Autodesk Inventor part; units mm, degrees
ref_plane "b_s_XY" through (11.5, 12, 6) normal (0, 0, 1) x (1, 0, 0)
ref_plane "b_s_YZ" through (11.5, 12, 6) normal (1, 0, 0) x (0, 1, 0)
ref_plane "b_s_ZX" through (11.5, 12, 6) normal (0, 1, 0) x (0, 0, 1)
sketch "Sketch_1" plane through (0, 0, 0) normal (0, 0, 1) x (1, 0, 0)
  line L0 (17, 0) -> (0, 0)
  line L1 (0, 18) -> (0, 6)
  line L2 (0, 6) -> (17, 6)
  line L3 (17, 6) -> (17, 18)
  line L4 (17, 18) -> (0, 18)
revolve "Revolution1" add sketch "Sketch_1" angle 360 about axis through (17, 0, 0) along (1, 0, 0)
sketch "Sketch_2" plane through (0, 0, 0) normal (0, 0, 1) x (1, 0, 0)
  line L0 (4.5, -5.8) -> (6, -5.8)
  line L1 (6, -5.8) -> (6, 30.2)
  line L2 (6, 30.2) -> (4.5, 30.2)
  line L3 (4.5, 30.2) -> (4.5, -5.8)
extrude "Extrusion1" cut sketch "Sketch_2" along normal mid plane 36
sketch "Sketch3" plane through (17, 0, 0) normal (1, 0, 0) x (0, 0, -1)
  point P0 (-12.5, 0)
hole "Hole1" at (17, 0, 12.5) direction (-1, 0, 0) diameter 5.5 depth 17 counterbore diameter 9.5 counterbore depth 12.5
sketch "Sketch4" plane through (17, 0, 0) normal (1, 0, 0) x (0, 0, -1)
  point P0 (12.5, 0)
hole "Hole2" at (17, 0, -12.5) direction (-1, 0, 0) diameter 5.5 depth 17 counterbore diameter 9.5 counterbore depth 12.5
sketch "Sketch_5" plane through (17, 0, 0) normal (1, 0, 0) x (0, 0, -1)
  line L0 (-0.75, 0) -> (0.75, 0)
  line L1 (0.75, 0) -> (0.75, 36)
  line L2 (0.75, 36) -> (-0.75, 36)
  line L3 (-0.75, 36) -> (-0.75, 0)
extrude "Extrusion2" cut sketch "Sketch_5" against normal blind 11
sketch "Sketch_6" plane through (0, 0, 0) normal (0, 0, 1) x (1, 0, 0)
  arc A0 (9.5, -6) -> (17, -14.4) centre (26.2631, 1.4189) ccw
  line L0 (17, -14.4) -> (17, 3.6)
  line L1 (17, 3.6) -> (9.5, 3.6)
  line L2 (9.5, 3.6) -> (9.5, -6)
extrude "Extrusion3" cut sketch "Sketch_6" along normal mid plane 1.5
sketch "Sketch_4" plane through (11.5, 0, 0) normal (1, 0, 0) x (0, 0, -1)
  line L0 (0, 12) -> (-18, 12)
  line L1 (-18, 12) -> (-18, 16.5)
  line L2 (-18, 16.5) -> (-6, 16.5)
  line L3 (-6, 16.5) -> (-6, 14.75)
  line L4 (-6, 14.75) -> (0, 14.75)
  line L5 (0, 14.75) -> (0, 12)
  line L6 (0, 12) -> (-18, 12)
revolve "Revolution2" cut sketch "Sketch_4" angle 360 about axis through (11.5, 12, 0) along (0, 0, -1)
sketch "Sketch_7" plane through (11.5, 0, 0) normal (1, 0, 0) x (0, 0, -1)
  line L0 (0.75, 12) -> (15.2889, 12)
  line L1 (15.2889, 12) -> (15.2889, 9.5)
  line L2 (15.2889, 9.5) -> (14.8559, 9.933)
  line L3 (14.8559, 9.933) -> (1.183, 9.933)
  line L4 (1.183, 9.933) -> (0.75, 9.5)
  line L5 (0.75, 9.5) -> (0.75, 12)
  line L6 (0.75, 12) -> (15.2889, 12)
revolve "Revolution3" cut sketch "Sketch_7" angle 360 about axis through (11.5, 12, -0.75) along (0, 0, 1)
thread "Thread1"
ref_plane "b_s_XY" through (11.5, 12, 6) normal (0, 0, 1) x (1, 0, 0)
ref_plane "b_s_YZ" through (11.5, 12, 6) normal (1, 0, 0) x (0, 1, 0)
ref_plane "b_s_ZX" through (11.5, 12, 6) normal (0, 1, 0) x (0, 0, 1)
properties part number "SSTHMR12b"
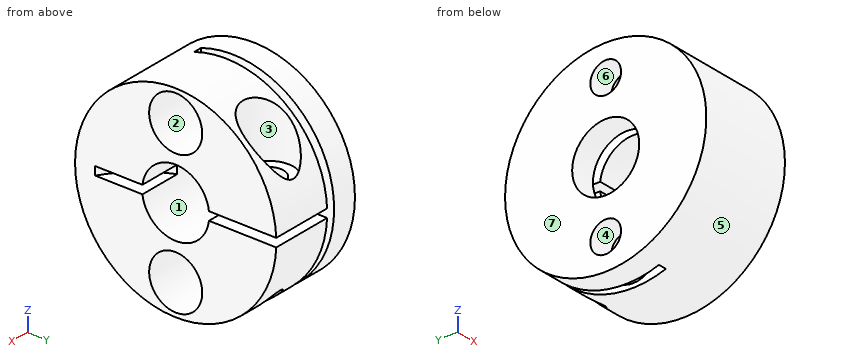
Model file for the job. Use its own axes, mm. Face numbers are marked on the shaded views. A direction names the side the tool comes from. Give positions to 0.01 mm unless a question says otherwise; leave off trailing zeros. Order: outer loops, then holes, each group sorted by start corner. A loop starts at its lowest first (then second) coordinate and runs counter-clockwise, first axis right, second up. Notation, with made-up numbers: M 85,-17.5 L 117,-17.5 A20 ccw 117,-5.5 Z; hole C 62.5,13.5 d2. An arc over 180 degrees is marked long. Put each result on its own line as item: value. Start each with the question number.
(1) Drill centre lines: L1, parallel to Z at x = 13.5, y = 0; L2, parallel to Z at x = 2.55, y = 0; L3, parallel to X at y = 12, z = 4.25. Where is each one in solid material? Low to high. Write a range as [from, to].
(2) Band-saw the part on B-B on z = -3.5. Give the cut face in (x, y).
(3) Band-saw the part on A-A on y = 0. Count the separate pieces of the cut face and the enclosed holes in it, then the cut area to 4 significant figures.
(4) Tool access for the marked faces 1, 2 and 3: list every direction of +Z, -Z, +X, -X, +Y, -Y with a clear straight run to the whole face (end or side of a thin tool).
(5) Pin check, flat tips, straight feed: pin 1 Ø8.5 at (x, y) = (12.5, -9) entering from -Z; pin 2 Ø6 at (x, y) = (10.5, -7) entering from +Z; pin 3 Ø4 at (x, z) = (11, -3) entering from +Y; pin 4 Ø5 at (y, z) = (0, -12.5) entering from -X. Stop position of each tip, or through.
(6) Band-saw the part on D-D on z = 12.5. Give the cut face in (x, y), then the cut area to 3 significant figures.
(7) Pull direction Z, two halves, no side cores. Call the marked faces 4, 5, 6 and 7: released by +Z, released by -Z, zero draft, split by the parting line, or undercut.
(8) Band-saw the part on C-C on y = 12. Give the cut face in (x, z).
Results below:
1. L1: z = [-18, -17.25], [-7.75, -6], [6, 7.75], [17.25, 18]
1. L2: z = [-18, -15.25], [-9.75, -6], [6, 9.75], [15.25, 18]
1. L3: x = [0, 4.5], [6, 8.75], [14.25, 17]
2. outline: M 0,-17.66 L 17,-17.66 L 17,-4.87 L 6,-4.87 L 6,-5.8 L 4.5,-5.8 L 4.5,-4.87 L 0,-4.87 Z; M 0,4.87 L 4.5,4.87 L 4.5,17.66 L 0,17.66 Z; M 6,4.87 L 17,4.87 L 17,17.66 L 6,17.66 Z; hole C 11.5,12 d4.13
3. separate pieces: 8
3. enclosed holes: 0
3. area: 113.5 mm2
4. face 1: +X, -X
4. face 2: +X
4. face 3: +Z
5. pin 1: stops at z = -17.36
5. pin 2: stops at z = 17.55
5. pin 3: stops at y = 17.97
5. pin 4: passes through
6. outline: M 0,-12.95 L 17,-12.95 L 17,-4.75 L 6,-4.75 L 6,-5.8 L 4.5,-5.8 L 4.5,-2.75 L 0,-2.75 Z; M 0,2.75 L 4.5,2.75 L 4.5,12.95 L 0,12.95 Z; M 6,4.75 L 17,4.75 L 17,12.95 L 15.9,12.95 A4.5 cw long 7.1,12.95 L 6,12.95 Z
6. area: 243 mm2
7. face 4: undercut
7. face 5: split by the parting line
7. face 6: undercut
7. face 7: zero draft
8. outline: M 0,-13.42 L 4.5,-13.42 L 4.5,13.42 L 0,13.42 Z; M 6,-13.42 L 9.43,-13.42 L 9.43,-1.18 L 9,-0.75 L 6,-0.75 Z; M 6,0.75 L 8.75,0.75 L 8.75,6 L 7,6 L 7,13.42 L 6,13.42 Z; M 13.57,-13.42 L 17,-13.42 L 17,-0.75 L 14,-0.75 L 13.57,-1.18 Z; M 14.25,0.75 L 17,0.75 L 17,13.42 L 16,13.42 L 16,6 L 14.25,6 Z
